Geometry: final body of the model. Coordinates: model frame, mm. A direction names the side the tool comes from. Give positions to 0.01 mm unless a question says otherwise; leave off trailing zeros. Write each loop counter-clockwise with the first axis right and the second up, starting at its lowest first coordinate (ties: lowest second). Pieces come first, ordered by that corner, then holes. Notation, with made-up numbers: (14, 35) -> (51, 35) arc R13 cw to (51, 52) -> close; hole circle Ø4 at (11, 63). An arc over 180 degrees is marked (long way). Use CSV: the item, a comma, the result in double quotes. Start each with the question number.
1) Material intervals for line 1 (Y direction, x = 15, z = 18.5); line 2 (Y direction, x = -5.1, z = 31.2); line 3 (Z direction, x = 3, y = 2.75), sorted ascending. Write a range as [from, to].
2) Section D-D (y = 4). Output: boundary loops of the cut face in (x, z).
3) Section C-C (x = 13.6). Output: boundary loops of the cut face in (y, z), plus the area to 3 significant figures.
4) Draft query along Z for faces 1 (the face through (-2, 0, 28.2)), 2 (the face through (12.6, 0, 19.1)), 3 (the face through (-11.1, 0, 9)). Return one class per face: pulls with the +Z half, pulls with the -Z half, needs draft (parallel to the pull), parting line crosses it, or undercut.
5) Section A-A (x = -13.6). Output: boundary loops of the cut face in (y, z).
6) Section B-B (x = 1.1). Output: boundary loops of the cut face in (y, z), plus the area to 3 significant figures.
7) Contact query for flat-ended pins moving along their axis: P1, Ø6, axis at y = -1.5, z = 7.5, coming from the +X side; P2, Ø3.5, axis at x = 4.5, y = 3, coming from the +Z side; P3, Ø1.2, axis at x = -13, y = -1, coming from the +Z side. Output: stop coordinate, or through.
8) Set-up query: faces 4 (the face through (-12.6, 0, 19.1)), 5 (the face through (-13.6, 2, 5.5)), 6 (the face through (-10, 5, 24.2)). Return all of +Z, -Z, +X, -X, +Y, -Y with unobstructed straight access to the full face (end or side cutting, diameter ignored); none if empty.
Autodesk Inventor part; units mm, degrees
ref_plane "YZ Plane" through (0, 0, 0) normal (1, 0, 0) x (0, 1, 0)
ref_plane "XZ Plane" through (0, 0, 0) normal (0, 1, 0) x (-1, 0, 0)
ref_plane "XY Plane" through (0, 0, 0) normal (0, 0, 1) x (1, 0, 0)
sketch "Sketch1" plane through (0, 0, 0) normal (0, 0, 1) x (1, 0, 0)
  line L0 (-11.1, 6) -> (11.1, 6)
  line L1 (11.1, 6) -> (11.1, -6)
  line L2 (11.1, -6) -> (-11.1, -6)
  line L3 (-11.1, -6) -> (-11.1, 6)
  point P0 (0, 0)
  dimension "d0" = 22.2
  dimension "d1" = 12
  dimension "d2" = 6
  dimension "d3" = 11.1
extrude "Extrusion1" add sketch "Sketch1" along normal blind 18
sketch "Sketch2" plane through (0, 0, 18) normal (0, 0, 1) x (1, 0, 0)
  line L0 (-16.1, 6) -> (16.1, 6)
  line L1 (16.1, 6) -> (16.1, -6)
  line L2 (16.1, -6) -> (-16.1, -6)
  line L3 (-16.1, -6) -> (-16.1, 6)
  line L4 (11.1, 6) -> (-11.1, 6)
  line L5 (-11.1, -6) -> (11.1, -6)
  line L6 (-11.1, 6) -> (-11.1, -6)
  line L7 (11.1, -6) -> (11.1, 6)
  point P0 (0, 0)
  dimension "d6" = 5
  dimension "d7" = 5
extrude "Extrusion2" add sketch "Sketch2" along normal blind 2.2
sketch "Sketch3" plane through (0, 0, 20.2) normal (0, 0, 1) x (1, 0, 0)
  line L0 (16.1, 6) -> (-16.1, 6)
  line L1 (-16.1, -6) -> (16.1, -6)
  line L2 (-11.1, 6) -> (11.1, 6)
  line L3 (11.1, 6) -> (11.1, -6)
  line L4 (11.1, -6) -> (-11.1, -6)
  line L5 (-11.1, -6) -> (-11.1, 6)
  line L6 (-16.1, 6) -> (-16.1, -6)
  line L7 (16.1, -6) -> (16.1, 6)
  point P0 (0, 0)
  point P1 (-11.1, -6)
  dimension "d10" = 5
  dimension "d11" = 5
extrude "Extrusion3" add sketch "Sketch3" along normal blind 4 contours L3 L1 L5 L0
sketch "Sketch4" plane through (0, 0, 24.2) normal (0, 0, 1) x (1, 0, 0)
  circle A0 centre (-5.1, 0) radius 6
  line L0 (11.1, 6) -> (-11.1, 6)
  line L1 (-11.1, 6) -> (-11.1, -6)
  point P0 (0, 0)
  dimension "d14" = 6
extrude "Extrusion4" add sketch "Sketch4" along normal blind 4 contours A0
sketch "Sketch5" plane through (0, 0, 24.2) normal (0, 0, 1) x (1, 0, 0)
  circle A0 centre (1.1, 0) radius 2.6
  line L0 (11.1, -6) -> (11.1, 6)
  point P0 (0, 0)
  dimension "d17" = 5.2
  dimension "d18" = 10
extrude "Extrusion5" add sketch "Sketch5" along normal blind 4
sketch "Sketch6" plane through (0, 0, 28.2) normal (0, 0, 1) x (1, 0, 0)
  arc A0 (0.3581, 2.4919) -> (0.3581, -2.4919) centre (-5.1, 0) ccw
  circle A1 centre (-5.1, 0) radius 2.2
  point P0 (0, 0)
  dimension "d21" = 4.4
extrude "Extrusion6" add sketch "Sketch6" along normal blind 4
sketch "Sketch7" plane through (-5.1, 0, 32.2) normal (0, 0, 1) x (1, 0, 0)
  point P0 (5.1, 0)
  point P1 (0, 0)
hole "Hole1" at (-5.1, 0, 32.2) direction (0, 0, -1) diameter 2 depth 4 tip angle 118
sketch "Sketch8" plane through (0, 0, 20.2) normal (0, 0, 1) x (1, 0, 0)
  line L0 (-16.1, 6) -> (-16.1, -6)
  line L1 (16.1, -6) -> (16.1, 6)
  point P0 (0, 0)
  point P1 (-13.6, 0)
  point P2 (13.6, 0)
  dimension "d31" = 2.5
  dimension "d32" = 2.5
hole "Hole2" at (-13.6, 0, 20.2) at (13.6, 0, 20.2) direction (0, 0, -1) diameter 2 depth 4 tip angle 118
sketch "Sketch9" plane through (0, 0, 20.2) normal (0, 0, 1) x (1, 0, 0)
  line L0 (-16.1, 6) -> (-16.1, -6)
  line L1 (-16.1, 0.5) -> (-14.0089, 0.5)
  line L2 (-14.0089, 0.5) -> (-14.0089, -0.5)
  line L3 (-14.0089, -0.5) -> (-16.1, -0.5)
  line L4 (-16.1, -0.5) -> (-16.1, 0.5)
  circle A0 centre (-13.6, 0) radius 1
  line L5 (16.1, -6) -> (16.1, 6)
  line L6 (13.947, 0.5) -> (16.1, 0.5)
  line L7 (16.1, 0.5) -> (16.1, -0.5)
  line L8 (16.1, -0.5) -> (13.947, -0.5)
  line L9 (13.947, -0.5) -> (13.947, 0.5)
  circle A1 centre (13.6, 0) radius 1
  point P0 (0, 0)
  point P1 (-14.466, -0.5)
  point P2 (-14.466, 0.5)
  dimension "d40" = 1
  dimension "d41" = 0.5
  dimension "d42" = 1
  dimension "d43" = 0.5
extrude "Extrusion7" cut sketch "Sketch9" against normal blind 4 contours L1 A0 L3 L0 | L8 A1 L6 L5 | L8 L9 L6 A1 picked at (14.1647, 0)
sketch "Sketch10" plane through (-11.1, -6, 0) normal (-1, 0, 0) x (0, 0, 1)
  line L0 (6, 8) -> (5, 8)
  line L1 (5, 8) -> (5, 4)
  line L2 (5, 4) -> (6, 4)
  line L3 (6, 4) -> (6, 8)
  line L4 (0, 12) -> (0, 0)
  line L5 (0, 0) -> (18, 0)
  line L6 (0, 12) -> (18, 12)
  point P0 (0, 6)
  dimension "d46" = 1
  dimension "d47" = 5
  dimension "d48" = 4
  dimension "d49" = 4
extrude "Extrusion8" add sketch "Sketch10" along normal blind 5
properties part number "mg90s-servo"
Answers follow:
1,line 1,"y = [-6, -0.5], [0.5, 6]"
1,line 2,"y = [-2.2, -1], [1, 2.2]"
1,line 3,"z = [0, 24.2]"
2,outline,"(-16.1, 18) -> (-11.1, 18) -> (-11.1, 0) -> (11.1, 0) -> (11.1, 18) -> (16.1, 18) -> (16.1, 20.2) -> (11.1, 20.2) -> (11.1, 24.2) -> (-0.63, 24.2) -> (-0.63, 28.2) -> (-9.57, 28.2) -> (-9.57, 24.2) -> (-11.1, 24.2) -> (-11.1, 20.2) -> (-16.1, 20.2) -> close"
3,outline,"(-6, 18) -> (-1, 18) -> (-1, 20.2) -> (-6, 20.2) -> close; (1, 18) -> (6, 18) -> (6, 20.2) -> (1, 20.2) -> close"
3,area,"22.0 mm^2"
4,face 1,"pulls with the +Z half"
4,face 2,"needs draft"
4,face 3,"undercut"
5,outline,"(-6, 18) -> (-1, 18) -> (-1, 20.2) -> (-6, 20.2) -> close; (-2, 5) -> (2, 5) -> (2, 6) -> (-2, 6) -> close; (1, 18) -> (6, 18) -> (6, 20.2) -> (1, 20.2) -> close"
6,outline,"(-6, 0) -> (6, 0) -> (6, 24.2) -> (2.6, 24.2) -> (2.6, 28.2) -> (-2.6, 28.2) -> (-2.6, 24.2) -> (-6, 24.2) -> close"
6,area,"311 mm^2"
7,P1,"stops at x = 11.1"
7,P2,"stops at z = 24.2"
7,P3,"stops at z = 20.2"
8,face 4,"+Z"
8,face 5,"-Z, -X, +Y"
8,face 6,"+Z, -X, +Y"
